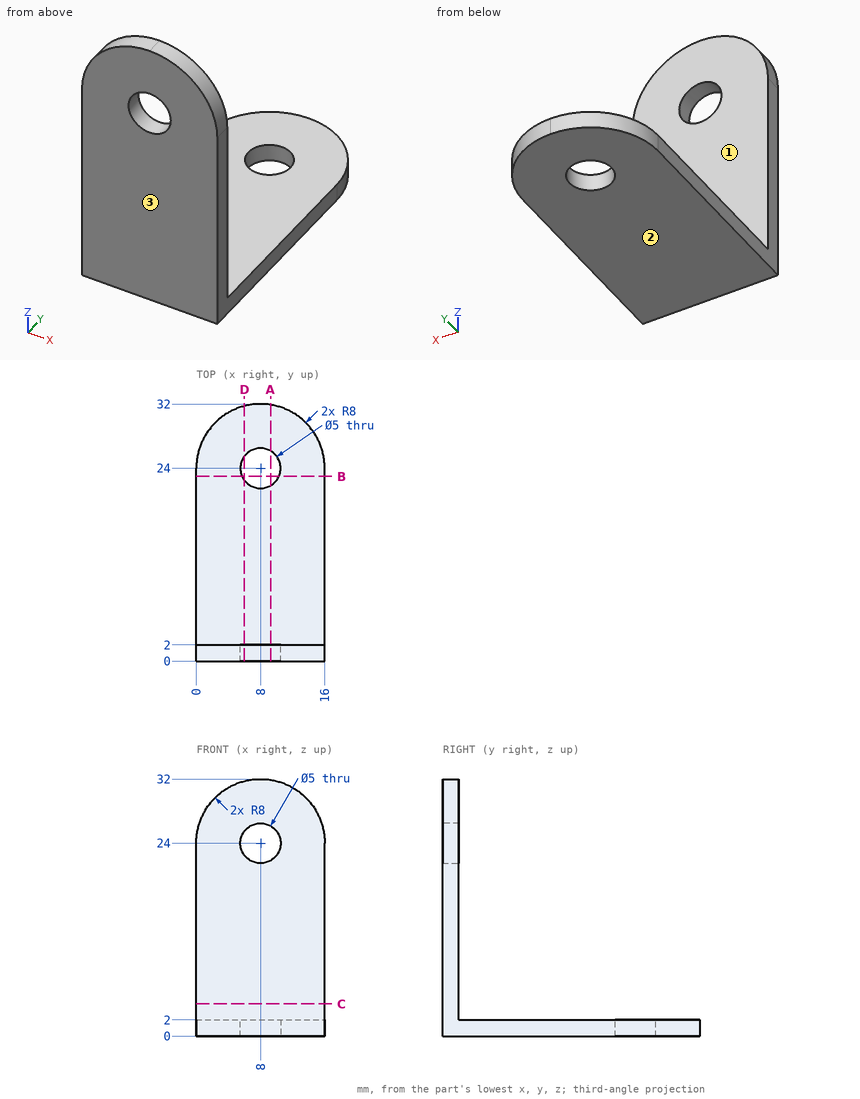
For this review, use the dimensioned drawing (mm, ordinates from the lowest corner) and the shaded views. Round coordinates to 2 decimals unless told otherwise and drop trailing zeros. Write each loop counter-clockwise with the first axis right and the second up, starting at its lowest first coordinate (ties: lowest second). Pieces come first, ordered by that corner, then holes. Notation, with made-up numbers: M 51.25,-39.75 L 82.25,-39.75 A11 cw 82.25,-23.75 Z; hole C 41,45.25 d8. An arc over 180 degrees is marked long. Use CSV: the item, a comma, the result in double quotes. Start each with the question number.
(1) We need section D-D, the plane x = 6. State the section outline as (y, z) points, then the cut area to 3 significant figures.
(2) We need section C-C, the plane z = 4. State the section outline as (x, y) points.
(3) We need section B-B, the plane y = 23. State the section outline as (x, z) points, then the cut area to 3 significant figures.
(4) Clearance check with flat-ended pins moving along their axes: P1, Ø4, axis at x = 6, z = 19.5, coming from the +Y side; P2, Ø4, axis at x = 3.5, y = 26.5, coming from the +Z side. State where each tip first meets the part, or that it passes through.
(5) We need section A-A, the plane x = 9.25. State the section outline as (y, z) points (3 decimals), then the cut area to 3 significant figures.
(6) The part is to be moulded in two halves that separate along Y. For the marked faces 1, 2 and 3, say which applies: +Y half, -Y half, draft (parallel to the pull), parting line (faces both ways), or undercut.
(7) For line 1 along X through (y, z) = (1, 24); line 2 along Z through (x, y) = (7.75, 31.5), list the stretches that pass through material, from the lowest coordinate up.
Findings:
1,outline,"M 0,0 L 22.5,0 L 22.5,2 L 2,2 L 2,22.5 L 0,22.5 Z; M 0,25.5 L 2,25.5 L 2,31.75 L 0,31.75 Z; M 25.5,0 L 31.75,0 L 31.75,2 L 25.5,2 Z"
1,area,"111 mm^2"
2,outline,"M 0,0 L 16,0 L 16,2 L 0,2 Z"
3,outline,"M 0,0 L 5.71,0 L 5.71,2 L 0,2 Z; M 10.29,0 L 16,0 L 16,2 L 10.29,2 Z"
3,area,"22.8 mm^2"
4,P1,"y = 2"
4,P2,"z = 2"
5,outline,"M 0,0 L 21.835,0 L 21.835,2 L 2,2 L 2,21.835 L 0,21.835 Z; M 0,26.165 L 2,26.165 L 2,31.902 L 0,31.902 Z; M 26.165,0 L 31.902,0 L 31.902,2 L 26.165,2 Z"
5,area,"106 mm^2"
6,face 1,"+Y half"
6,face 2,"draft"
6,face 3,"-Y half"
7,line 1,"0 to 5.5, 10.5 to 16"
7,line 2,"0 to 2"
